Design review of the part built by this model. Coordinates are the model's own, in mm. A direction names the side the tool comes from. Coordinates: 2 decimals unless noted, no trailing zeros. Order: outer loops, then holes, each group sorted by start corner. A loop starts at its lowest first (then second) coordinate and runs counter-clockwise, first axis right, second up. Notation, with made-up numbers: M 76,61 L 99,61 A29 cw 99,100 Z; hole C -18.75,-33.75 d6. An arc over 180 degrees is marked long. Use CSV: the item, a comma, the result in double quotes.
```python
from build123d import *

# Parameters (mm, degrees)
F1_DEPTH  = 254
F2_W      = 254
F2_H      = 1016
F3_DEPTH  = 508
F5_DEPTH  = 309.88
F7_DEPTH  = 508
F9_DEPTH  = 254
F10_W     = 254
F10_H     = 254
F11_DEPTH = 254
F13_DEPTH = 254
F15_DEPTH = 254
F17_DEPTH = 254


with BuildPart() as f1:
    # F0 (on Front) → F1 (new body)
    with BuildSketch(Plane.XZ):
        Polygon((1524, 508), (0, 508), (0, -762), (762, -762), (762, 0), (1524, 0), align=None)
    extrude(amount=F1_DEPTH)

    # F2 (on face) → F3 (join)
    with BuildSketch(Plane.XZ.offset(254)):
        with Locations((127, -254)):
            Rectangle(F2_W, F2_H)
    extrude(amount=F3_DEPTH)

    # F4 (on face) → F5 (cut)
    with BuildSketch(Plane(origin=(0, 0, 0), x_dir=(0, -1, 0), z_dir=(-1, 0, 0))):
        Polygon((762, 254), (254, -762), (508, -762), (762, -762), align=None)
    extrude(amount=-F5_DEPTH, mode=Mode.SUBTRACT)

    # F6 (on face) → F7 (join)
    with BuildSketch(Plane.XZ.offset(254)):
        Polygon((1524, 508), (0, 508), (0, 254), (254, 254), (1524, 254), align=None)
    extrude(amount=F7_DEPTH)

    # F8 (on face) → F9 (cut)
    with BuildSketch(Plane.XZ.offset(762)):
        Polygon((762, 508), (508, 508), (508, 254), (1270, 254), (1270, 508), (1016, 508), align=None)
    extrude(amount=-F9_DEPTH, mode=Mode.SUBTRACT)

    # F10 (on face) → F11 (join)
    with BuildSketch(Plane.XZ.offset(762)):
        with Locations((1397, 381)):
            Rectangle(F10_W, F10_H)
    extrude(amount=F11_DEPTH)

    # F12 (on face) → F13 (cut)
    with BuildSketch(Plane.XZ.offset(254)):
        with BuildLine():
            ThreePointArc((762, -508), (687.605122, -687.605122), (508, -762))
            Line((508, -762), (762, -762))
            Line((762, -762), (762, -508))
        make_face()
    extrude(amount=-F13_DEPTH, mode=Mode.SUBTRACT)

    # F14 (on face) → F15 (cut)
    with BuildSketch(Plane.XZ.offset(254)):
        with BuildLine():
            Line((1524, 0), (1524, 254))
            ThreePointArc((1524, 254), (1449.605122, 74.394878), (1270, 0))
            Line((1270, 0), (1524, 0))
        make_face()
    extrude(amount=-F15_DEPTH, mode=Mode.SUBTRACT)

    # F16 (on face) → F17 (cut)
    with BuildSketch(Plane(origin=(0, 0, 254), x_dir=(1, 0, 0), z_dir=(0, 0, -1))):
        with BuildLine():
            Line((1524, 1016), (1270, 1016))
            ThreePointArc((1270, 1016), (1449.605122, 941.605122), (1524, 762))
            Line((1524, 762), (1524, 1016))
        make_face()
    extrude(amount=-F17_DEPTH, mode=Mode.SUBTRACT)


solid = f1.part
```
(1) The part is to be moulded in two halves that separate along X. For faces 4 (the face through (689.57, -128.78, -685.62)), 5 (the face through (884, -508, 383)), 6 (the face through (0, -291, 23)), say which applies: pulls with the +X half, pulls with the -X half, needs draft (parallel to the pull), parting line crosses it, or undercut.
The answers:
face 4,"pulls with the +X half"
face 5,"undercut"
face 6,"pulls with the -X half"
(2) Add section A-A on y = -687.5. State the section outline as (x, z) points.
The answers:
outline,"M 0,105 L 254,105 L 254,254 L 508,254 L 508,508 L 0,508 Z; M 1270,254 L 1524,254 L 1524,508 L 1270,508 Z"
(3) Add section D-D on y = -574.5. State the section outline as (x, z) points.
The answers:
outline,"M 0,-121 L 254,-121 L 254,254 L 508,254 L 508,508 L 0,508 Z; M 1270,254 L 1524,254 L 1524,508 L 1270,508 Z"
(4) Add section C-C on x = 1094. State the section outline as (y, z) points, and give its area (3 significant figures).
The answers:
outline,"M -508,254 L -254,254 L -254,0 L 0,0 L 0,508 L -508,508 Z"
area,"194,000 mm2"
(5) For faces 1 (the face through (250, -762, 383)), 2 (the face through (254, -392, -35)), 3 (the face through (1012, -125, 0)), list the 3-axis set-ups (+Z, -Z, +X, -X, +Y, -Y) from which the entire face can be reached by the end or side of a thin tool; tool diameter is ignored.
The answers:
face 1,"+Z, -Z, -X, -Y"
face 2,"-Z, +X, -Y"
face 3,"-Z, +X, +Y, -Y"
(6) Add section B-B on z = -99.5. State the section outline as (x, y) points, and give its area (3 significant figures).
The answers:
outline,"M 0,-585.25 L 254,-585.25 L 254,-254 L 762,-254 L 762,0 L 0,0 Z"
area,"278,000 mm2"
(7) Wall thickness on probe 1 along Z at (x, y) = (1418.5, -521); probe 2 along Y at (x, z) = (385, -407.5); probe 3 along X at (y, z) = (-670.5, 385): over which ranges is each line inside the solid? List them lowest first.
The answers:
probe 1,"z = 254 to 508"
probe 2,"y = -254 to 0"
probe 3,"x = 0 to 508, 1270 to 1524"
(8) Clearance check with flat-ended pins moving along their axes: P1, Ø8, axis at x = 271, z = -290.5, coming from the +Y side; P2, Ø6, axis at y = -317, z = -209.5, coming from the +X side. State where each tip first meets the part, or that it passes through.
The answers:
P1,"stops at y = 0"
P2,"stops at x = 254"
